from build123d import *

# Parameters (mm, degrees)
SKETCH4_W           = 31.05
SKETCH4_H           = 18.35
BOSS_EXTRUDE1_DEPTH = 19
SHELL1_T            = 2
SKETCH5_W           = 12
SKETCH5_H           = 18.35
CUT_EXTRUDE1_DEPTH  = 2


with BuildPart() as part:
    # Sketch4 → Boss-Extrude1 (new body)
    with BuildSketch(Plane(origin=(0, 0, 0), x_dir=(0, 0, -1), z_dir=(1, 0, 0))):
        Rectangle(SKETCH4_W, SKETCH4_H)
    extrude(amount=BOSS_EXTRUDE1_DEPTH)

    # Shell1
    shell1_openings = [part.faces().sort_by_distance(p)[0] for p in [
        (0, 0, 0),
    ]]
    offset(amount=SHELL1_T, openings=shell1_openings, kind=Kind.INTERSECTION)

    # Sketch5 → Cut-Extrude1 (cut)
    with BuildSketch(Plane(origin=(0, 0, -17.525), x_dir=(-1, 0, 0), z_dir=(0, 0, -1))):
        with Locations((-6, 0)):
            Rectangle(SKETCH5_W, SKETCH5_H)
    extrude(amount=-CUT_EXTRUDE1_DEPTH, mode=Mode.SUBTRACT)


solid = part.part
Input: part model. Units: mm. Frame: model coordinates. A direction names the side the tool comes from. Give positions to 0.01 mm unless a question says otherwise; leave off trailing zeros. Loops run counter-clockwise (first coordinate to the right, second up) from the corner with the lowest first, then second, coordinate; pieces in that order, holes last. Notation, with made-up numbers: (40.25, -10) -> (92.25, -10) arc R21 cw to (92.25, 1) -> close; hole circle Ø4 at (35.5, -7). An arc over 180 degrees is marked (long way). Answer as a JSON object with one key per item and string values. Group by question number.
Item 1: Cut plane C-C, the plane x = 5.75. Return the cut outline in (y, z) (3 decimals).
Item 2: Pin query (flat end, axial travel): P1, Ø9, axis at x = 5.5, y = 0, coming from the -Z side (3 decimals); P2, Ø1.6, axis at y = -2.5, z = -17, coming from the -X side; P3, Ø9, axis at y = 2.5, z = 6.5, coming from the -X side. Return the tip coordinate at first contact, or that it passes through.
Item 3: Line query: probe 1 along Y at (x, z) = (11.5, 7.5) (3 decimals); probe 2 along Z at (x, y) = (15.5, -6.75) (3 decimals); probe 3 along Z at (x, y) = (3.75, -3.5) (3 decimals). Output: solid intervals per line, ascending.
Item 4: Cut plane A-A, the plane x = 17.5. Return the cut outline in (y, z) (3 decimals), and give its area (3 significant figures).
Item 5: Pull-direction query (Z, two-part tool) for faces 1 (the flat face through (10, 0, 17.525)), 2 (the flat face through (9, 0, 15.525)), 3 (the flat face through (21, 0, 0)); classes: released by +Z, released by -Z, zero draft, split by the parting line, or undercut.
Item 6: Reachability of faces 4 (the flat face through (15, 0, -17.525)), 5 (the flat face through (12, 0, -17)), 6 (the flat face through (19, 0, 0)) from +Z, -Z, +X, -X, +Y, -Y: full face, straight path, thin tool, end or side. Return the list, or none.
Item 7: Cut plane B-B, the plane z = 2. Return the cut outline in (x, y) (3 decimals), and give its area (3 significant figures).
Checks:
{
 "1": {"outline": "(-11.175, -17.525) -> (-9.175, -17.525) -> (-9.175, 15.525) -> (9.175, 15.525) -> (9.175, -17.525) -> (11.175, -17.525) -> (11.175, 17.525) -> (-11.175, 17.525) -> close"},
 "2": {"P1": "stops at z = 15.525", "P2": "stops at x = 12", "P3": "stops at x = 19"},
 "3": {"probe 1": "y = -11.175 to -9.175, 9.175 to 11.175", "probe 2": "z = -17.525 to -15.525, 15.525 to 17.525", "probe 3": "z = 15.525 to 17.525"},
 "4": {"outline": "(-11.175, -17.525) -> (11.175, -17.525) -> (11.175, 17.525) -> (-11.175, 17.525) -> close; hole (-9.175, -15.525) -> (9.175, -15.525) -> (9.175, 15.525) -> (-9.175, 15.525) -> close", "area": "214 mm²"},
 "5": {"face 1": "released by +Z", "face 2": "undercut", "face 3": "zero draft"},
 "6": {"face 4": "-Z, +X, -X, +Y, -Y", "face 5": "-Z, -X", "face 6": "-X"},
 "7": {"outline": "(0, -11.175) -> (21, -11.175) -> (21, 11.175) -> (0, 11.175) -> (0, 9.175) -> (19, 9.175) -> (19, -9.175) -> (0, -9.175) -> close", "area": "121 mm²"}
}
